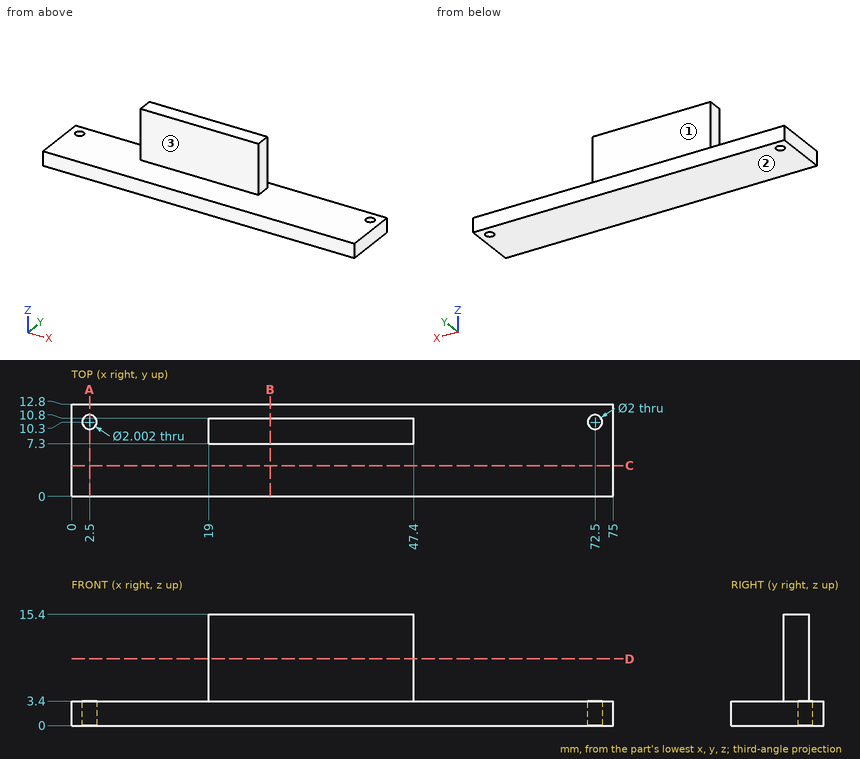
Geometry check sheet. Reference: drawing and pictorial views, mm from the part's lowest x, y, z. A direction names the side the tool comes from. Round coordinates to 2 decimals unless told otherwise and drop trailing zeros. Order: outer loops, then holes, each group sorted by start corner. A loop starts at its lowest first (then second) coordinate and runs counter-clockwise, first axis right, second up. Notation, with made-up numbers: M -39,89 L 13,89 A20 cw 13,112 Z; hole C 7,-37.75 d9. An arc over 180 degrees is marked long. Answer in a Markdown table with one row per item.
(1) Go/stop test with flat-tipped pins: P1, Ø6, axis at x = 27, z = 8.5, coming from the -Y side; P2, Ø4, axis at x = 17.5, y = 3, coming from the +Z side; P3, Ø1, axis at y = 8.5, z = 8.5, coming from the -X side; P4, Ø1.6, axis at x = 2.5, y = 10.3, coming from the -Z side. Record where each tip stops, or that it passes through.
Responses:
| item | result |
|---|---|
| P1 | stops at y = 7.3 |
| P2 | stops at z = 3.4 |
| P3 | stops at x = 19 |
| P4 | passes through |
(2) Sectioned sample at C-C, the plane y = 4.25. Record the cut outline in (x, z).
Responses:
| item | result |
|---|---|
| outline | M 0,0 L 75,0 L 75,3.4 L 0,3.4 Z |
(3) Scan lines: probe 1 along X at (y, z) = (11, 2.75) (1 decimal); probe 2 along Y at (x, z) = (2.5, 2.2); probe 3 along Z at (x, y) = (27, 11.75). Record each from-to range of solid material in increasing order. Write a range as from..to.
Responses:
| item | result |
|---|---|
| probe 1 | x = 0..1.8, 3.2..71.8, 73.2..75 |
| probe 2 | y = 0..9.3, 11.3..12.8 |
| probe 3 | z = 0..3.4 |
(4) Sectioned sample at D-D, the plane z = 9.25. Record the cut outline in (x, y), and give its area (3 significant figures).
Responses:
| item | result |
|---|---|
| outline | M 19,7.3 L 47.4,7.3 L 47.4,10.8 L 19,10.8 Z |
| area | 99.4 mm² |
(5) Sectioned sample at B-B, the plane x = 27.5. Record the cut outline in (y, z).
Responses:
| item | result |
|---|---|
| outline | M 0,0 L 12.8,0 L 12.8,3.4 L 10.8,3.4 L 10.8,15.4 L 7.3,15.4 L 7.3,3.4 L 0,3.4 Z |
(6) Tool access check on the marked faces 1, 2 and 3. Record the directions out of +Z, -Z, +X, -X, +Y, -Y that give a thin tool (end or side, any length) a straight path to the whole face; none if there is none.
Responses:
| item | result |
|---|---|
| face 1 | +Z, +X, -X, +Y |
| face 2 | -Z, +X, -X, +Y, -Y |
| face 3 | +Z, +X, -X, -Y |
(7) Sectioned sample at A-A, the plane x = 2.5. Record the cut outline in (y, z).
Responses:
| item | result |
|---|---|
| outline | M 0,0 L 9.3,0 L 9.3,3.4 L 0,3.4 Z; M 11.3,0 L 12.8,0 L 12.8,3.4 L 11.3,3.4 Z |
